Geometry: final body of the model. Coordinates: model frame, mm. A direction names the side the tool comes from. Round coordinates to 2 decimals unless told otherwise and drop trailing zeros. Loops run counter-clockwise (first coordinate to the right, second up) from the corner with the lowest first, then second, coordinate; pieces in that order, holes last. Notation, with made-up numbers: (-7, -31) - (29, -31) arc R19 cw to (29, -4) - close; hole circle Ø11 at (79.25, -6.75). An arc over 180 degrees is marked (long way). Return JSON: item names as keys, results as strings. Group by question number.
1. Material intervals for probe 1 along X at (y, z) = (-4.5, -23.75); probe 2 along X at (y, z) = (11.5, -30); probe 3 along Y at (x, z) = (-32, -19.25), sorted ascending.
2. Draft query along Z for faces 1 (the face through (-24, 14, -22)), 2 (the face through (-18.4, 13.39, -15.17)), 3 (the face through (-19.097, 14.771, -14.902)), 4 (the face through (-20, 12, -27)). Return one class per face: +Z half, -Z half, draft (parallel to the pull), parting line (faces both ways), or undercut.
3. Section C-C on z = -12. Return loops of the section in (x, y), and give its area (3 significant figures).
4. Set-up query: faces 5 (the face through (-25, 14, -8)), 6 (the face through (-18.924, 16.346, -15.168)), 7 (the face through (-22.8, 0.4, -17)), 8 (the face through (-23.468, 21.637, -15.168)), 9 (the face through (-31.5, 21.77, -15.17)). Return all of +Z, -Z, +X, -X, +Y, -Y with unobstructed straight access to the full face (end or side cutting, diameter ignored); none if empty.
5. Section A-A on y = -8.5. Return loops of the section in (x, z).
6. Section D-D on x = -28.5. Return loops of the section in (y, z).
7. First-contact query: pin 1 Ø4.5 at (x, y) = (-30, 22) entering from -Z; pin 2 Ø10.5 at (x, y) = (-22.5, -6.5) entering from +Z; pin 3 Ø8 at (x, z) = (-26.5, -11.5) entering from +Y; pin 4 Ø1.8 at (y, z) = (19.5, -29) entering from -X. Flat tips, straight axial feed; report the tip coordinate or a pass-through.
8. Section B-B on z = -23. Return loops of the section in (x, y).
Autodesk Inventor part; units mm, degrees
ref_plane "YZ Plane" through (0, 0, 0) normal (1, 0, 0) x (0, 1, 0)
ref_plane "XZ Plane" through (0, 0, 0) normal (0, 1, 0) x (-1, 0, 0)
ref_plane "XY Plane" through (0, 0, 0) normal (0, 0, 1) x (1, 0, 0)
sketch "Sketch1" plane through (0, 0, 0) normal (0, 1, 0) x (-1, 0, 0)
  line L0 (0, 0) -> (26, 0)
  line L1 (26, 0) -> (26, -33)
  line L2 (26, -33) -> (0, -33)
  line L3 (0, -33) -> (0, 0)
  dimension "d0" = 26
  dimension "d1" = 33
extrude "Extrusion1" add sketch "Sketch1" along normal blind 4
sketch "Sketch2" plane through (0, 0, 0) normal (0, -1, 0) x (1, 0, 0)
  line L0 (-26, 0) -> (0, 0)
  line L1 (-26, -33) -> (-26, 0)
  line L2 (0, -33) -> (-26, -33)
  line L3 (0, 0) -> (0, -33)
  line L4 (-26, 0) -> (0, 0)
  line L5 (-26, -33) -> (-26, 0)
  line L6 (0, 0) -> (0, -33)
  line L7 (0, -33) -> (-26, -33)
  line L8 (0, 0) -> (-4, 0)
  line L9 (-4, 0) -> (-4, -33)
  line L10 (-4, -33) -> (0, -33)
  line L11 (0, -33) -> (0, 0)
  line L12 (-26, -33) -> (-26, 0)
  line L13 (-26, 0) -> (-23, 0)
  line L14 (-23, 0) -> (-23, -33)
  line L15 (-23, -33) -> (-26, -33)
  line L16 (-26, -33) -> (-26, 0)
  dimension "d4" = 4
  dimension "d5" = 3
extrude "Extrusion2" add sketch "Sketch2" along normal blind 17 contours L0 L14 L2 L1 | L0 L3 L2 L9
sketch "Sketch3" plane through (0, 4, 0) normal (0, 1, 0) x (1, 0, 0)
  line L0 (0, 33) -> (-26, 33)
  line L1 (-26, 33) -> (-26, 0)
  line L2 (-26, 0) -> (0, 0)
  line L3 (0, 0) -> (0, 33)
  line L4 (0, 0) -> (-6, 0)
  line L5 (-6, 0) -> (-6, 33)
  line L6 (-6, 33) -> (0, 33)
  line L7 (0, 33) -> (0, 0)
  line L8 (-6, 33) -> (-26, 33)
  line L9 (-26, 33) -> (-26, 27)
  line L10 (-26, 27) -> (-6, 27)
  line L11 (-6, 27) -> (-6, 33)
  dimension "d8" = 6
  dimension "d9" = 6
extrude "Extrusion3" add sketch "Sketch3" along normal blind 10 contours L5 L10 L1 L0
sketch "Sketch4" plane through (-26, 4, -27) normal (0, 0, 1) x (1, 0, 0)
  line L0 (20, 0) -> (0, 0)
  line L1 (20, 0) -> (20, 10)
  line L2 (0, 10) -> (20, 10)
  line L3 (0, 0) -> (0, 10)
  line L4 (20, 10) -> (6, 10)
  line L5 (6, 10) -> (6, 7)
  line L6 (6, 7) -> (20, 7)
  line L7 (20, 7) -> (20, 10)
  line L8 (20, 7) -> (6, 7)
  line L9 (6, 7) -> (6, 1)
  line L10 (6, 1) -> (20, 1)
  line L11 (20, 1) -> (20, 7)
  point P0 (26, -4)
  dimension "d12" = 14
  dimension "d13" = 3
  dimension "d14" = 6
sketch "Sketch5" plane through (0, 14, 0) normal (0, 1, 0) x (1, 0, 0)
  line L0 (-6, 27) -> (-6, 33)
  line L1 (-6, 33) -> (-26, 33)
  line L2 (-26, 33) -> (-26, 27)
  line L3 (-26, 27) -> (-6, 27)
  line L4 (-26, 33) -> (-6, 33)
  line L5 (-6, 33) -> (-6, 27)
  line L6 (-6, 27) -> (-26, 27)
  line L7 (-26, 27) -> (-26, 33)
  point P0 (0, 0)
extrude "Extrusion4" add sketch "Sketch5" along normal blind 12
sketch "Sketch6" plane through (-26, 4, -27) normal (0, 0, 1) x (1, 0, 0)
  line L0 (20, 0) -> (20, 22)
  line L1 (20, 22) -> (4.2431, 19.2216)
  line L2 (20, 22) -> (36, 22) construction
  line L3 (4.2431, 19.2216) -> (4.764, 16.2672)
  line L4 (4.764, 16.2672) -> (20.5209, 19.0456)
  line L5 (20.5209, 19.0456) -> (20, 22)
  line L6 (4.764, 16.2672) -> (5.8059, 10.3584)
  line L7 (5.8059, 10.3584) -> (6.3269, 7.4039)
  line L8 (6.3269, 7.4039) -> (22.0838, 10.1823)
  line L9 (22.0838, 10.1823) -> (21.5628, 13.1367)
  line L10 (21.5628, 13.1367) -> (5.8059, 10.3584)
  line L11 (20, 0) -> (0, 0)
  line L12 (20, 0) -> (20, 22)
  line L13 (0, 22) -> (20, 22)
  line L14 (0, 0) -> (0, 22)
  line L15 (0, -21) -> (0, 22)
  line L16 (20, 22) -> (10, 22)
  line L17 (20, 22) -> (0, 22)
  line L18 (10, 22) -> (-5.7569, 19.2216)
  line L19 (10, 22) -> (26, 22) construction
  line L20 (-5.7569, 19.2216) -> (-5.236, 16.2672)
  line L21 (-5.236, 16.2672) -> (10.5209, 19.0456)
  line L22 (10.5209, 19.0456) -> (10, 22)
  line L23 (-5.236, 16.2672) -> (-4.1941, 10.3584)
  line L24 (-5.236, 16.2672) -> (0.764, 16.2672) construction
  line L25 (-4.1941, 10.3584) -> (11.5628, 13.1367)
  line L26 (11.5628, 13.1367) -> (10.5209, 19.0456)
  line L27 (-4.1941, 10.3584) -> (-3.6731, 7.4039)
  line L28 (-4.1941, 10.3584) -> (-1.1941, 10.3584) construction
  line L29 (-3.6731, 7.4039) -> (12.0838, 10.1823)
  line L30 (12.0838, 10.1823) -> (11.5628, 13.1367)
  point P0 (26, -4)
  dimension "d17" = 16
  dimension "d18" = 170
  dimension "d19" = 3
  dimension "d20" = 6
  dimension "d21" = 3
  dimension "d22" = 16
  dimension "d27" = 16
  dimension "d28" = 170
  dimension "d29" = 16
  dimension "d30" = 6
  dimension "d31" = 80
  dimension "d32" = 3
  dimension "d33" = 80
  dimension "d34" = 16
extrude "Extrusion5" add sketch "Sketch6" along normal blind 24 contours L29 L27 L25 L14 | L14 L25 L6 L7 L29 | L30 L29 L7 L10 | L10 L6 L25 L30 | L21 L20 L18 L14 | L14 L18 L22 L1 L3 L21 | L22 L21 L3 L1
sketch "Sketch7" plane through (-26, 4, 0) normal (0, 0, 1) x (1, 0, 0)
  line L0 (3, -4) -> (22, -4)
  line L1 (22, -4) -> (22, -21)
  line L2 (26, -21) -> (22, -21)
  line L3 (26, -21) -> (26, 0)
  line L4 (0, 0) -> (26, 0)
  line L5 (0, -21) -> (0, 0)
  line L6 (3, -21) -> (0, -21)
  line L7 (3, -4) -> (3, -21)
  line L8 (0, -21) -> (3, -21)
  line L9 (20, 0) -> (0, 0)
  line L10 (3, -21) -> (0, -21)
  line L11 (0, -21) -> (0, 0)
  line L12 (0, 0) -> (3, 0)
  line L13 (3, 0) -> (3, -21)
  line L14 (26, -4) -> (0, -4)
  line L15 (0, -4) -> (0, 0)
  line L16 (0, 0) -> (26, 0)
  line L17 (26, 0) -> (26, -4)
  line L18 (22, -4) -> (22, -21)
  line L19 (26, -4) -> (22, -4)
  line L20 (22, -4) -> (22, -21)
  line L21 (22, -21) -> (26, -21)
  line L22 (26, -21) -> (26, -4)
extrude "Extrusion6" cut sketch "Sketch7" against normal blind 17
sketch "Sketch8" plane through (-26, 4, -27) normal (0, 0, 1) x (1, 0, 0)
  line L0 (11.5628, 13.1367) -> (-4.1941, 10.3584)
  line L1 (-4.1941, 10.3584) -> (-3.6731, 7.4039)
  line L2 (-3.6731, 7.4039) -> (12.0838, 10.1823)
  line L3 (12.0838, 10.1823) -> (11.5628, 13.1367)
  line L4 (12.0838, 10.1823) -> (0, 8.0516)
  line L5 (0, 0) -> (0, 8.0516)
  line L6 (20, 0) -> (0, 0)
  line L7 (20, 0) -> (20, 22)
  line L8 (10, 22) -> (20, 22)
  line L9 (10, 22) -> (10.5209, 19.0456)
  line L10 (10.5209, 19.0456) -> (0, 17.1905)
  line L11 (0, 11.0979) -> (0, 17.1905)
  line L12 (0, 11.0979) -> (11.5628, 13.1367)
  line L13 (11.5628, 13.1367) -> (12.0838, 10.1823)
  point P0 (26, -4)
sketch "Sketch9" plane through (-26, -17, -33) normal (-1, 0, 0) x (0, 0, 1)
  line L0 (16, 0) -> (16, 21)
  line L1 (6, 21) -> (16, 21)
  line L2 (6, 21) -> (6, 29.0516)
  line L3 (6, 29.0516) -> (6, 32.0979)
  line L4 (6, 32.0979) -> (6, 38.1905)
  line L5 (6, 38.1905) -> (6, 41.2367)
  line L6 (6, 41.2367) -> (6, 43)
  line L7 (0, 43) -> (6, 43)
  line L8 (0, 0) -> (0, 43)
  line L9 (16, 0) -> (0, 0)
  line L10 (0, 17) -> (0, 0)
  line L11 (16, 21) -> (0, 21)
  line L12 (0, 21) -> (0, 0)
  line L13 (0, 0) -> (16, 0)
  line L14 (16, 0) -> (16, 21)
  point P0 (33, 17)
sketch "Sketch10" plane through (-4, -17, -33) normal (-1, 0, 0) x (0, 0, 1)
  line L0 (16, 0) -> (16, 17)
  line L1 (0, 17) -> (16, 17)
  line L2 (0, 17) -> (0, 0)
  line L3 (16, 0) -> (0, 0)
  line L4 (16, 17) -> (0, 17)
  line L5 (0, 17) -> (0, 0)
  line L6 (0, 0) -> (16, 0)
  line L7 (16, 0) -> (16, 17)
  point P0 (33, 17)
sketch "Sketch11" plane through (-23, -17, -33) normal (1, 0, 0) x (0, 0, -1)
  line L0 (-16, 17) -> (-16, 0)
  line L1 (0, 0) -> (-16, 0)
  line L2 (0, 17) -> (0, 0)
  line L3 (-16, 17) -> (0, 17)
  line L4 (-16, 17) -> (0, 17)
  line L5 (0, 17) -> (0, 0)
  line L6 (0, 0) -> (-16, 0)
  line L7 (-16, 0) -> (-16, 17)
  point P0 (-33, 17)
sketch "Sketch12" plane through (0, -17, -33) normal (1, 0, 0) x (0, 0, -1)
  line L0 (-16, 21) -> (-16, 0)
  line L1 (0, 0) -> (-16, 0)
  line L2 (0, 21) -> (0, 0)
  line L3 (-16, 21) -> (0, 21)
  line L4 (0, 17) -> (-16, 17)
  line L5 (-16, 21) -> (0, 21)
  line L6 (0, 21) -> (0, 0)
  line L7 (0, 0) -> (-16, 0)
  line L8 (-16, 0) -> (-16, 21)
  point P0 (-33, 17)
extrude "Extrusion7" add sketch "Sketch10" along normal blind 10
extrude "Extrusion8" cut sketch "Sketch12" against normal blind 10
extrude "Extrusion9" add sketch "Sketch9" along normal blind 10 contours L9 L8 L11 L1 L0
extrude "Extrusion10" cut sketch "Sketch11" against normal blind 10
sketch "Sketch13" plane through (-26, 4, -17) normal (0, 0, 1) x (1, 0, 0)
  point P0 (26, -4)
sketch "Sketch15" plane through (-13.9162, 14.1823, -27) normal (0.1736482, -0.9848078, 0) x (0.9848078, 0.1736482, 0)
  line L0 (-16, 0) -> (-12.2702, 0)
  line L1 (0, 0) -> (-12.2702, 0)
  line L2 (0, 0) -> (0, 24)
  line L3 (-16, 24) -> (0, 24)
  line L4 (-16, 0) -> (-16, 24)
  line L5 (-16, 0) -> (-16, 5)
  line L6 (-16, 24) -> (-16, 19)
  line L7 (-16, 24) -> (-11, 24) construction
  line L8 (-16, 19) -> (-5, 19)
  line L9 (-5, 19) -> (-5, 5)
  line L10 (-5, 5) -> (-16, 5)
  line L11 (-16, 5) -> (-16, 19)
  point P0 (11.2421, 27)
  dimension "d43" = 5
  dimension "d44" = 5
  dimension "d45" = 90
  dimension "d46" = 11
extrude "Extrusion11" cut sketch "Sketch15" against normal blind 4 contours L4 L8 L9 L10
sketch "Sketch16" plane through (-6, 26, -27) normal (1, 0, 0) x (0, 0, -1)
  point P0 (-27, -26)
sketch "Sketch17" plane through (-6, 26, -27) normal (1, 0, 0) x (0, 0, -1)
  line L0 (6, -22) -> (0, -22)
  line L1 (6, -22) -> (6, 0)
  line L2 (0, 0) -> (6, 0)
  line L3 (0, -22) -> (0, 0)
  line L4 (0, 0) -> (6, 0)
  line L5 (6, 0) -> (6, -22)
  line L6 (6, -22) -> (0, -22)
  line L7 (0, -22) -> (0, 0)
  point P0 (-27, -26)
extrude "Extrusion12" cut sketch "Sketch17" against normal blind 7.5
properties part number "HolderMagasin_3DPrint"
Taken from the geometry:
{
 "1": {"probe 1": "-36 to -33, -14 to -10", "probe 2": "-26 to -13.5", "probe 3": "0 to 4"},
 "2": {"face 1": "undercut", "face 2": "draft", "face 3": "undercut", "face 4": "+Z half"},
 "3": {"outline": "(-31.76, 23.22) - (-31.24, 20.27) - (-15.48, 23.05) - (-16, 26) - close; (-19.36, 16.27) - (-18.84, 13.31) - (-13.92, 14.18) - (-14.44, 17.14) - close", "area": "63.0 mm2"},
 "4": {"face 5": "-X, -Y", "face 6": "+Z, -X", "face 7": "+Z, +X, -X, -Y", "face 8": "+Z, +X", "face 9": "+Z, -Z, -X"},
 "5": {"outline": "(-36, -33) - (-33, -33) - (-33, -17) - (-36, -17) - close; (-14, -33) - (-10, -33) - (-10, -17) - (-14, -17) - close"},
 "6": {"outline": "(0, -33) - (4, -33) - (4, -17) - (0, -17) - close; (11.61, -27) - (14.66, -27) - (14.66, -22) - (11.61, -22) - close; (11.61, -8) - (14.66, -8) - (14.66, -3) - (11.61, -3) - close; (20.75, -27) - (23.8, -27) - (23.8, -3) - (20.75, -3) - close"},
 "7": {"pin 1": "z = -27", "pin 2": "through", "pin 3": "y = 24.85", "pin 4": "x = -26"},
 "8": {"outline": "(-36, -17) - (-33, -17) - (-33, 0) - (-14, 0) - (-14, -17) - (-10, -17) - (-10, 4) - (-36, 4) - close; (-31.76, 23.22) - (-31.24, 20.27) - (-15.48, 23.05) - (-16, 26) - close; (-30.19, 14.36) - (-29.67, 11.4) - (-13.92, 14.18) - (-14.44, 17.14) - close"}
}
